Autodesk Inventor part; units mm, degrees
ref_plane "YZ Plane" through (0, 0, 0) normal (1, 0, 0) x (0, 1, 0)
ref_plane "XZ Plane" through (0, 0, 0) normal (0, 1, 0) x (-1, 0, 0)
ref_plane "XY Plane" through (0, 0, 0) normal (0, 0, 1) x (1, 0, 0)
sketch "Sketch1" plane through (0, 0, 0) normal (0, 1, 0) x (-1, 0, 0)
  line L0 (0, 0) -> (50, 0)
  line L1 (50, 0) -> (50, -50)
  line L2 (50, -50) -> (0, -50)
  line L3 (0, -50) -> (0, 0)
  dimension "d0" = 50
  dimension "d1" = 50
extrude "Extrusion1" add sketch "Sketch1" along normal blind 2
fillet "Fillet1" radius 2 4 edges at (0, 1, 0) (0, 1, -50) (-50, 1, 0) (-50, 1, -50)
sketch "Sketch2" plane through (0, 2, 0) normal (0, 1, 0) x (1, 0, 0)
  line L0 (-48, 2) -> (-2, 2) construction
  line L1 (-2, 2) -> (-2, 48) construction
  line L2 (-2, 48) -> (-48, 48) construction
  line L3 (-48, 48) -> (-48, 2) construction
  line L4 (-48, 0) -> (-2, 0)
  line L5 (-50, 48) -> (-50, 2)
  line L6 (-2, 50) -> (-48, 50)
  line L7 (0, 2) -> (0, 48)
  line L8 (-25, 2) -> (-25, 6) construction
  line L9 (-25, 4) -> (-20, 4)
  line L10 (-20, 4) -> (-20, 6)
  line L11 (-20, 6) -> (-30, 6)
  line L12 (-30, 6) -> (-30, 4)
  line L13 (-30, 4) -> (-25, 4)
  line L14 (-48, 25) -> (-46, 25) construction
  line L15 (-46, 25) -> (-46, 20)
  line L16 (-46, 20) -> (-48, 20)
  line L17 (-46, 25) -> (-46, 30)
  line L18 (-46, 30) -> (-48, 30)
  line L19 (-48, 20) -> (-48, 30)
  line L20 (-4, 25) -> (-4, 20)
  line L21 (-4, 20) -> (-2, 20)
  line L22 (-4, 25) -> (-4, 30)
  line L23 (-4, 30) -> (-2, 30)
  line L24 (-2, 20) -> (-2, 30)
  line L25 (-25, 48) -> (-25, 44) construction
  line L26 (-25, 46) -> (-20, 46)
  line L27 (-20, 46) -> (-20, 44)
  line L28 (-20, 44) -> (-30, 44)
  line L29 (-30, 44) -> (-30, 46)
  line L30 (-30, 46) -> (-25, 46)
  point P0 (0, 0)
  dimension "d5" = 2
  dimension "d6" = 2
  dimension "d7" = 2
  dimension "d8" = 2
  dimension "d9" = 4
  dimension "d10" = 5
  dimension "d11" = 10
  dimension "d12" = 2
  dimension "d13" = 5
  dimension "d14" = 5
extrude "Extrusion2" add sketch "Sketch2" along normal blind 2 contours L15 L16 L19 L18 L17 | L22 L23 L24 L21 L20
extrude "Extrusion3" add sketch "Sketch2" along normal blind 4.1 contours L13 L12 L11 L10 L9 | L26 L27 L28 L29 L30
sketch "Sketch3" plane through (-20, 2, -46) normal (0, 0, -1) x (-1, 0, 0)
  line L0 (10, 4.1) -> (0, 4.1)
  line L1 (0, 4.1) -> (10, 4.1)
  line L2 (10, 4.1) -> (10, 2.1)
  line L3 (10, 2.1) -> (0, 2.1)
  line L4 (0, 2.1) -> (0, 4.1)
  point P0 (-20, -2)
  dimension "d19" = 10
  dimension "d20" = 2
extrude "Extrusion4" add sketch "Sketch3" along normal blind 2
fillet "Fillet2" radius 0.5 1 edges at (-25, 4.1, -48)
ref_plane "Work Plane1" through (-46, 4, -25) normal (0, 0, -1) x (1, 0, 0)
mirror "Mirror1" about plane through (-46, 4, -25) normal (0, 0, -1) of "Extrusion4"
fillet "Fillet3" radius 0.5 1 edges at (-25, 4.1, -2)
fillet "Fillet4" radius 0.5 7 edges at (-2, 4, -25) (-4, 4, -25) (-46, 4, -25) (-48, 4, -25) (-25, 6.1, -2) (-25, 6.1, -6) (-25, 6.1, -44)
sketch "Sketch4" plane through (0, 2, 0) normal (0, 1, 0) x (1, 0, 0)
  line L0 (-30, 2.5) -> (-20, 2.5)
  line L1 (-25, 2.5) -> (-25, 49.5156) construction
  line L2 (-30, 46) -> (-20, 46)
  line L3 (-11, 11) -> (-39, 11)
  line L4 (-39, 11) -> (-39, 29)
  line L5 (-39, 29) -> (-11, 29)
  line L6 (-11, 29) -> (-11, 11)
  line L7 (-11, 11) -> (-39, 29) construction
  line L8 (-39, 11) -> (-11, 29) construction
  line L9 (-48, 0) -> (-2, 0)
  point P0 (0, 0)
  point P1 (-25, 20)
  dimension "d26" = 28
  dimension "d27" = 18
  dimension "d28" = 20
extrude "Extrusion5" cut sketch "Sketch4" against normal blind 2
fillet "Fillet5" radius 1 4 edges at (-39, 1, -11) (-11, 1, -11) (-11, 1, -29) (-39, 1, -29)
properties part number "180caseTop"
Source: CAD feature listing. Evaluate the final solid. Frame: model axes, mm. A direction names the side the tool comes from. Coordinates: 2 decimals unless noted, no trailing zeros. Order: outer loops, then holes, each group sorted by start corner. A loop starts at its lowest first (then second) coordinate and runs counter-clockwise, first axis right, second up. Notation, with made-up numbers: M 67,55 L 104,55 A28 cw 104,89 Z; hole C 70.25,85.5 d2. An arc over 180 degrees is marked long. Write each question's results on one line, items separated by ' | '. Start each with the question number.
1) Line query: line 1 (X direction, y = 1, z = -12); line 2 (Z direction, x = -33, y = 0.5); line 3 (Y direction, x = -28, z = -3). Output: solid intervals per line, ascending. Write a range as from..to.
2) Section query B-B (z = -16). Return the cut outline in (x, y).
3) Contact query for flat-ended pins moving along their axis: pin 1 Ø0.6 at (x, y) = (-3.5, 3.5) entering from -Z; pin 2 Ø0.5 at (x, z) = (-47, -24) entering from +Y; pin 3 Ø0.8 at (y, z) = (3, -23) entering from -X. Output: stop coordinate, or through.
4) Access query for faces 1 (the face through (-25, 3, -4)), 2 (the face through (-47, 3, -30)), 3 (the face through (-30, 4.5, -4.5)), 4 (the face through (-25, 3, -46)). Directions: +Z, -Z, +X, -X, +Y, -Y. A direction counts if a zero-diameter tool reaches every point of the face in a straight line with its end or side. Return the directions, or none.
5) Draft query along Z for faces 5 (the face through (-25, 1, -11)), 6 (the face through (-0.57, 1.01, -49.4)), 7 (the face through (-39, 1, -20)), 8 (the face through (-25, 6.1, -46)). Return one class per face: released by +Z, released by -Z, zero draft, split by the parting line, or undercut.
6) Section query C-C (y = 1). Return the cut outline in (x, z).
7) Section query D-D (x = -23.5). Return the cut outline in (y, z), plus the area to 3 significant figures.
8) Section query A-A (x = -31.5). Return the cut outline in (y, z), plus the area to 3 significant figures.
Answers:
1) line 1: x = -50..-39, -11..0 | line 2: z = -50..-29, -11..0 | line 3: y = 0..2, 4.1..6.1
2) outline: M -50,0 L -39,0 L -39,2 L -50,2 Z; M -11,0 L 0,0 L 0,2 L -11,2 Z
3) pin 1: stops at z = -30 | pin 2: stops at y = 4 | pin 3: stops at x = -48
4) face 1: +Z, +X, -X | face 2: -Z, +X, -X, +Y | face 3: +Z, -Z, -X, +Y | face 4: -Z, +X, -X
5) face 5: undercut | face 6: released by -Z | face 7: undercut | face 8: zero draft
6) outline: M -50,-48 A2 ccw -48,-50 L -2,-50 A2 ccw 0,-48 L 0,-2 A2 ccw -2,0 L -48,0 A2 ccw -50,-2 Z; hole M -39,-28 A1 ccw -38,-29 L -12,-29 A1 ccw -11,-28 L -11,-12 A1 ccw -12,-11 L -38,-11 A1 ccw -39,-12 Z
7) outline: M 0,-50 L 2,-50 L 2,-46 L 4.1,-46 L 4.1,-47.5 A0.5 ccw 4.6,-48 L 6.1,-48 L 6.1,-44.5 A0.5 ccw 5.6,-44 L 2,-44 L 2,-29 L 0,-29 Z; M 0,-11 L 2,-11 L 2,-6 L 5.6,-6 A0.5 ccw 6.1,-5.5 L 6.1,-2.5 A0.5 ccw 5.6,-2 L 4.6,-2 A0.5 ccw 4.1,-2.5 L 4.1,-4 L 2,-4 L 2,0 L 0,0 Z | area: 88.1 mm^2
8) outline: M 0,-50 L 2,-50 L 2,-29 L 0,-29 Z; M 0,-11 L 2,-11 L 2,0 L 0,0 Z | area: 64.0 mm^2
